```python
from build123d import *

# Parameters (mm, degrees)
BOSS_EXTRUDE1_DEPTH = 4.9276
SKETCH2_R           = 5.355070432
BOSS_EXTRUDE2_DEPTH = 0.4953
FILLET1_R           = 10.16
SKETCH6_R           = 3.8989
BOSS_EXTRUDE3_DEPTH = 165.1


with BuildPart() as part:
    # Sketch1 → Boss-Extrude1 (new body)
    with BuildSketch(Plane.XY):
        Polygon((6.305518095, 0), (3.152759047, 5.460738854), (-3.152759047, 5.460738854), (-6.305518095, 0), (-3.152759047, -5.460738854), (3.152759047, -5.460738854), align=None)
    extrude(amount=BOSS_EXTRUDE1_DEPTH)

    # Sketch2 → Boss-Extrude2 (add)
    with BuildSketch(Plane.XY.offset(4.9276)):
        Circle(SKETCH2_R)
    extrude(amount=BOSS_EXTRUDE2_DEPTH)

    # Fillet1
    # the kernel refuses this fillet: 10.16 mm, written as the material it takes off along each edge
    with BuildSketch(Plane(origin=(0, 0, 5.4229), x_dir=(1, 0, 0), z_dir=(0, -1, 0))) as fillet1_piece_1:
        with BuildLine():
            CenterArc((2.22151432, -10.16), FILLET1_R, 72.035909036, 17.964090964)
            Line((2.22151432, 0), (2.22151432, 0.2032))
            Line((2.22151432, 0.2032), (5.355070432, 0.2032))
            Line((5.355070432, 0.2032), (5.558270432, 0))
            ThreePointArc((5.558270432, 0), (5.558270432, -0.24765), (5.417741555, -0.302006))
            Line((5.417741555, -0.302006), (5.355070432, -0.4953))
        make_face()
    revolve(axis=Axis((0, 0, 5.4229), (0, 0, 1)), mode=Mode.SUBTRACT)

    # Sketch6 → Boss-Extrude3 (add)
    with BuildSketch(Plane.XY.offset(5.4229)):
        Circle(SKETCH6_R)
    extrude(amount=BOSS_EXTRUDE3_DEPTH)


solid = part.part
```
Geometry: final body of the model. Coordinates: model frame, mm. A direction names the side the tool comes from. Give positions to 0.01 mm unless a question says otherwise; leave off trailing zeros. Order: outer loops, then holes, each group sorted by start corner. A loop starts at its lowest first (then second) coordinate and runs counter-clockwise, first axis right, second up. Notation, with made-up numbers: (67, 20) -> (123, 20) arc R24 cw to (123, 55) -> close; hole circle Ø1 at (34.25, -5.5). An arc over 180 degrees is marked (long way). Write each question's results on one line, items separated by ' | '. Start each with the question number.
1) Set-up query: faces 1 (the flat face through (6, 0, 4.928)), 2 (the flat face through (-4.751, -2.692, 2.429)). Return all of +Z, -Z, +X, -X, +Y, -Y with unobstructed straight access to the full face (end or side cutting, diameter ignored); none if empty.
2) First-contact query: pin 1 (6 mm diameter, centred on x = 0, z = 146, fed in from -Y); pin 2 (5 mm diameter, centred on y = 1, z = 78, fed in from +X); pin 3 (5 mm diameter, centred on x = 0.5, z = 139.5, fed in from +Y). Flat tips, straight axial feed; report the tip coordinate or a pass-through.
3) Section A-A (z = 133). Return loops of the section in (x, y), then the cut area to 3 significant figures.
4) Line query: line 1 (X direction, y = -0.25, z = 20); line 2 (X direction, y = -2.25, z = 50). Output: solid intervals per line, ascending. Write a range as from..to.
Calculated:
1) face 1: +Z | face 2: +Z, -Z, -X, -Y
2) pin 1: y = -3.9 | pin 2: x = 3.9 | pin 3: y = 3.9
3) outline: circle Ø7.8 at (0, 0) | area: 47.8 mm2
4) line 1: -3.89..3.89 | line 2: -3.18..3.18
